```python
from build123d import *

# Parameters (mm, degrees)
F0_W     = 12.7
F0_H     = 12.7
F1_DEPTH = 1.5875
F2_R     = 1.016
F2_R_2   = 1.397
F3_DEPTH = 6.35
F2_R_3   = 2.54
F4_DEPTH = 3.175
F5_DEPTH = 0.635


with BuildPart() as f1:
    # F0 (on Top) → F1 (new body)
    with BuildSketch(Plane.XY):
        Rectangle(F0_W, F0_H)
    extrude(amount=F1_DEPTH)

    # F2 (on face) → F3 (cut)
    with BuildSketch(Plane.XY.offset(1.5875)):
        with Locations((-3.175, 3.175)):
            Circle(F2_R)
        with Locations((3.175, -3.175)):
            Circle(F2_R)
        with Locations((-3.175, -3.175)):
            Circle(F2_R_2)
    extrude(amount=-F3_DEPTH, mode=Mode.SUBTRACT)

    # F2 (on face) → F4 (join)
    with BuildSketch(Plane.XY.offset(1.5875)):
        with Locations((3.175, -3.175)):
            Circle(F2_R_3)
        with Locations((3.175, -3.175)):
            Circle(F2_R, mode=Mode.SUBTRACT)
    extrude(amount=F4_DEPTH)

    # F2 (on face) → F5 (cut)
    with BuildSketch(Plane.XY.offset(1.5875)):
        with Locations((-3.175, -3.175)):
            Circle(F2_R_3)
        with Locations((-3.175, -3.175)):
            Circle(F2_R_2, mode=Mode.SUBTRACT)
    extrude(amount=-F5_DEPTH, mode=Mode.SUBTRACT)


solid = f1.part
```
The listing builds one solid part. Answer for the finished solid, in the listing's coordinates (mm). A direction names the side the tool comes from. Round coordinates to 2 decimals unless told otherwise and drop trailing zeros. Loops run counter-clockwise (first coordinate to the right, second up) from the corner with the lowest first, then second, coordinate; pieces in that order, holes last. Notation, with made-up numbers: (-35, 37.25) - (0, 37.25) arc R26 cw to (0, 61.25) - close; hole circle Ø1 at (12.5, 22). An arc over 180 degrees is marked (long way). Return JSON: item names as keys, results as strings. Group by question number.
1. Which of the six approach directions +Z, -Z, +X, -X, +Y, -Y give full straight-line access (tool end or side, diameter ignored) to faces 1 (the cylindrical face through (-0.83, -4.15, 1.27)), 2 (the cylindrical face through (-4.3, -4, 0.5))?
2. Consider probe 1 along Y at (x, z) = (3.25, 0.2); probe 2 along Z at (x, y) = (-4.5, 1.25); probe 3 along Z at (x, y) = (-2.25, -1). Determine where each line is inside the solid, lowest interval first.
3. The mould has two halves that part along X. Classify faces 3 (the flat face through (-2.1, -4.3, 0.952)), 4 (the flat face through (0, 0, 0)), 5 (the flat face through (-6.35, 0, 1)): pulls with the +X half, pulls with the -X half, needs draft (parallel to the pull), parting line crosses it, or undercut.
4. The part is cut by section A-A on y = -2.75. Determine the outline of the cut face in (x, z).
5. The part is cut by section C-C on y = 4. Determine the outline of the cut face in (x, z).
6. The part is cut by section D-D on x = 0. Determine the outline of the cut face in (y, z), then the cut area to 3 significant figures.
7. The part is cut by section B-B on x = 4. Determine the outline of the cut face in (y, z), then the cut area to 3 significant figures.
8. Each of these flat-tipped pins is pushed along its axis until it touches: P1, Ø1.5, axis at x = 3, y = 3.5, coming from the +Z side; P2, Ø4, axis at x = -3.175, y = -3.175, coming from the +Z side. Where does it stop, or does it pass through?
Resolved:
{
 "1": {"face 1": "+Z", "face 2": "+Z, -Z"},
 "2": {"probe 1": "y = -6.35 to -4.19, -2.16 to 6.35", "probe 2": "z = 0 to 1.59", "probe 3": "z = 0 to 0.95"},
 "3": {"face 3": "undercut", "face 4": "needs draft", "face 5": "pulls with the -X half"},
 "4": {"outline": "(-6.35, 0) - (-4.51, 0) - (-4.51, 0.95) - (-5.68, 0.95) - (-5.68, 1.59) - (-6.35, 1.59) - close; (-1.84, 0) - (2.25, 0) - (2.25, 4.76) - (0.67, 4.76) - (0.67, 1.59) - (-0.67, 1.59) - (-0.67, 0.95) - (-1.84, 0.95) - close; (4.1, 0) - (6.35, 0) - (6.35, 1.59) - (5.68, 1.59) - (5.68, 4.76) - (4.1, 4.76) - close"},
 "5": {"outline": "(-6.35, 0) - (-3.77, 0) - (-3.77, 1.59) - (-6.35, 1.59) - close; (-2.58, 0) - (6.35, 0) - (6.35, 1.59) - (-2.58, 1.59) - close"},
 "6": {"outline": "(-6.35, 0) - (6.35, 0) - (6.35, 1.59) - (-6.35, 1.59) - close", "area": "20.2 mm²"},
 "7": {"outline": "(-6.35, 0) - (-3.77, 0) - (-3.77, 4.76) - (-5.58, 4.76) - (-5.58, 1.59) - (-6.35, 1.59) - close; (-2.58, 0) - (6.35, 0) - (6.35, 1.59) - (-0.77, 1.59) - (-0.77, 4.76) - (-2.58, 4.76) - close", "area": "29.8 mm²"},
 "8": {"P1": "stops at z = 1.59", "P2": "stops at z = 0.95"}
}
